Could you check a few things on this model? Use its own coordinates, in mm. Face numbers are marked on the shaded views. A direction names the side the tool comes from. Round coordinates to 2 decimals unless told otherwise and drop trailing zeros. Loops run counter-clockwise (first coordinate to the right, second up) from the corner with the lowest first, then second, coordinate; pieces in that order, holes last. Notation, with made-up numbers: (23, -21) - (33, -21) arc R30 ccw to (33, 14) - close; hole circle Ø7 at (48, -2). An arc over 180 degrees is marked (long way). Use one line per item in the form item = value.
```python
from build123d import *

# Parameters (mm, degrees)
BOSS_EXTRUDE3_DEPTH = 15
BOSS_EXTRUDE4_DEPTH = 9.5
BOSS_EXTRUDE5_DEPTH = 13
FILLET2_R           = 2.5
FILLET3_R           = 2.5
SKETCH2_W           = 6.5
SKETCH2_H           = 11.5
CUT_EXTRUDE1_DEPTH  = 171.414201286


with BuildPart() as part:
    # Sketch1 → Boss-Extrude3 (new, symmetric)
    with BuildSketch(Plane(origin=(0, 0, 0), x_dir=(1, 0, 0), z_dir=(0, 1, 0))):
        Polygon((0, 61), (0, 35), (109.5, 35), (109.5, 48), (109.5, 61), align=None)
    extrude(amount=BOSS_EXTRUDE3_DEPTH, both=True)

    # Sketch1_7 → Boss-Extrude4 (add, symmetric)
    # profile 1 of 2: a face of its own
    with BuildSketch(Plane(origin=(0, 0, 0), x_dir=(1, 0, 0), z_dir=(0, 1, 0))):
        Polygon((0, 35), (0, 0), (105, 0), (105, 17), (133, 17), (115, 35), (109.5, 35), align=None)
        with BuildLine():
            ThreePointArc((30.5, 12), (25, 17.5), (30.5, 23))
            Line((30.5, 23), (81.5, 23))
            ThreePointArc((81.5, 23), (87, 17.5), (81.5, 12))
            Line((81.5, 12), (30.5, 12))
        make_face(mode=Mode.SUBTRACT)
    # profile 2 of 2: a face of its own
    with BuildSketch(Plane(origin=(0, 0, 0), x_dir=(1, 0, 0), z_dir=(0, 1, 0))):
        Polygon((0, 96), (0, 61), (109.5, 61), (115, 61), (133, 79), (105, 79), (105, 96), align=None)
        with BuildLine():
            Line((81.5, 73), (30.5, 73))
            ThreePointArc((30.5, 73), (25, 78.5), (30.5, 84))
            Line((30.5, 84), (81.5, 84))
            ThreePointArc((81.5, 84), (87, 78.5), (81.5, 73))
        make_face(mode=Mode.SUBTRACT)
    extrude(amount=BOSS_EXTRUDE4_DEPTH, both=True)

    # Sketch1_8 → Boss-Extrude5 (add, symmetric)
    with BuildSketch(Plane(origin=(0, 0, 0), x_dir=(1, 0, 0), z_dir=(0, 1, 0))):
        Polygon((105, 17), (105, 0), (140, 0), (140, 10), (133, 17), align=None)
        Polygon((140, 96), (105, 96), (105, 79), (133, 79), (140, 86), align=None)
    extrude(amount=BOSS_EXTRUDE5_DEPTH, both=True)

    # Fillet2
    fillet2_edges = [part.edges().sort_by_distance(p)[0] for p in [
        (87, 9.5, -17.5),
        (56, 9.5, -12),
        (25, 9.5, -17.5),
        (56, -9.5, -23),
        (56, 9.5, -23),
        (87, -9.5, -17.5),
        (25, -9.5, -17.5),
        (56, -9.5, -12),
    ]]
    fillet(fillet2_edges, radius=FILLET2_R)

    # Fillet3
    fillet3_edges = [part.edges().sort_by_distance(p)[0] for p in [
        (56, -9.5, -84),
        (87, -9.5, -78.5),
        (56, 9.5, -73),
        (25, -9.5, -78.5),
        (56, 9.5, -84),
        (87, 9.5, -78.5),
        (25, 9.5, -78.5),
        (56, -9.5, -73),
    ]]
    fillet(fillet3_edges, radius=FILLET3_R)

    # Sketch2 → Cut-Extrude1 (cut, through all)
    with BuildSketch(Plane.XY):
        with Locations((3.25, -9.25)):
            Rectangle(SKETCH2_W, SKETCH2_H)
    extrude(amount=-CUT_EXTRUDE1_DEPTH, mode=Mode.SUBTRACT)


solid = part.part
```
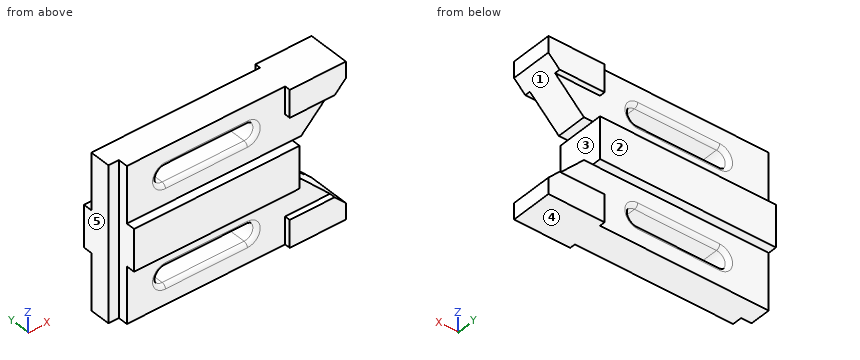
1. For P1, Ø3, axis at x = 58, y = 12, coming from the +Z side; P2, Ø5, axis at x = 125, z = -85.5, coming from the +Y side; P3, Ø4.5, axis at x = 52.5, y = -12.5, coming from the -Z side; P4, Ø8, axis at x = 20, y = 7.5, coming from the +Z side, each with a flat end and sliding along its axis, tell me the tip position at first contact or that it passes through.
Solution:
P1 = -35
P2 = 13
P3 = -61
P4 = 0
2. Please list where these lines run through material, in increasing order: line 1 along Z through (x, y) = (75.5, -1.5); line 2 along Z through (x, y) = (108, -11.25); line 3 along Z through (x, y) = (127, 0).
Solution:
line_1 = -96 to -84, -73 to -23, -12 to 0
line_2 = -96 to -79, -61 to -35, -17 to 0
line_3 = -96 to -73, -23 to 0
3. If we section it at C-C, the plane x = 10.5: Write out the boundary of the cut face in (y, z).
Solution:
outline = (-15, -61) - (-9.5, -61) - (-9.5, -96) - (9.5, -96) - (9.5, -61) - (15, -61) - (15, -35) - (9.5, -35) - (9.5, 0) - (-9.5, 0) - (-9.5, -35) - (-15, -35) - close
4. If we section it at B-B, the plane y = 5.25: Write out the boundary of the cut face in (x, z), plus the area to 3 significant figures.
Solution:
outline = (0, -96) - (140, -96) - (140, -86) - (115, -61) - (109.5, -61) - (109.5, -35) - (115, -35) - (140, -10) - (140, 0) - (0, 0) - close; hole (30.5, -84) - (81.5, -84) arc R5.5 ccw to (81.5, -73) - (30.5, -73) arc R5.5 ccw to start; hole (30.5, -23) - (81.5, -23) arc R5.5 ccw to (81.5, -12) - (30.5, -12) arc R5.5 ccw to start
area = 10,700 mm^2
5. On a 3-axis mill with a long thin cutter (end or side, diameter ignored), from which of +Z, -Z, +X, -X, +Y, -Y can I reach the whole of each face in a straight line? I mean the marked faces 1 and 2. Say none if no direction works.
Solution:
face_1 = +X, +Y, -Y
face_2 = +Z, -Z, +X, -X, +Y
6. If we section it at D-D, the plane z = -64: Write out the boundary of the cut face in (x, y).
Solution:
outline = (0, -3.5) - (6.5, -3.5) - (6.5, -9.5) - (118, -9.5) - (118, 9.5) - (0, 9.5) - close
7. If we section it at A-A, the plane x = 63: Write out the boundary of the cut face in (y, z), plus the area to 3 significant figures.
Solution:
outline = (-15, -61) - (-9.5, -61) - (-9.5, -70.5) arc R2.5 ccw to (-7, -73) - (7, -73) arc R2.5 ccw to (9.5, -70.5) - (9.5, -61) - (15, -61) - (15, -35) - (9.5, -35) - (9.5, -25.5) arc R2.5 ccw to (7, -23) - (-7, -23) arc R2.5 ccw to (-9.5, -25.5) - (-9.5, -35) - (-15, -35) - close; (-9.5, -96) - (9.5, -96) - (9.5, -86.5) arc R2.5 ccw to (7, -84) - (-7, -84) arc R2.5 ccw to (-9.5, -86.5) - close; (-9.5, -9.5) arc R2.5 ccw to (-7, -12) - (7, -12) arc R2.5 ccw to (9.5, -9.5) - (9.5, 0) - (-9.5, 0) - close
area = 1,680 mm^2
8. We'd pull the mould along Z, two halves only. Please class the marked faces 3, 4 and 5: +Z half, -Z half, draft (parallel to the pull), parting line (faces both ways), or undercut.
Solution:
face_3 = undercut
face_4 = -Z half
face_5 = draft
